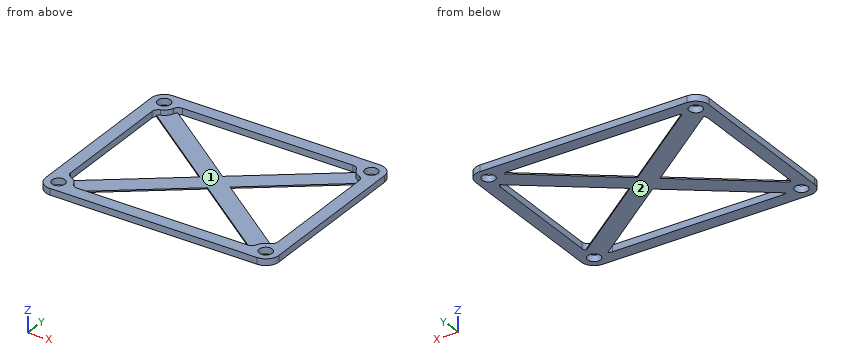
from build123d import *

# Parameters (mm, degrees)
SKETCH1_R           = 6.35
OUTLINE_DEPTH       = 6.35
FILLET2_R           = 12.7
BOSS_EXTRUDE1_DEPTH = 1.27
FILLET1_R           = 6.35


with BuildPart() as part:
    # Sketch1 → Outline (new body)
    with BuildSketch(Plane.XY):
        with BuildLine():
            Line((-101.6, 114.3), (101.6, 114.3))
            ThreePointArc((101.6, 114.3), (110.580256121, 110.580256121), (114.3, 101.6))
            Line((114.3, 101.6), (114.3, -66.802))
            Line((114.3, -66.802), (-114.3, -66.802))
            Line((-114.3, -66.802), (-114.3, 101.6))
            ThreePointArc((-114.3, 101.6), (-110.580256121, 110.580256121), (-101.6, 114.3))
        make_face()
        with Locations((-101.6, 101.6)):
            Circle(SKETCH1_R, mode=Mode.SUBTRACT)
        with Locations((101.6, 101.6)):
            Circle(SKETCH1_R, mode=Mode.SUBTRACT)
        with Locations((-101.6, -54.102)):
            Circle(SKETCH1_R, mode=Mode.SUBTRACT)
        with Locations(Location((101.6, -54.102, 0), (0, 0, 180))):
            Circle(SKETCH1_R, mode=Mode.SUBTRACT)
        with BuildLine():
            Line((-101.6, 88.9), (-101.6, -41.402))
            ThreePointArc((-101.6, -41.402), (-92.619743879, -45.121743879), (-88.9, -54.102))
            Line((-88.9, -54.102), (88.9, -54.102))
            ThreePointArc((88.9, -54.102), (92.619743879, -45.121743879), (101.6, -41.402))
            Line((101.6, -41.402), (101.6, 88.9))
            ThreePointArc((101.6, 88.9), (92.619743879, 92.619743879), (88.9, 101.6))
            Line((88.9, 101.6), (-88.9, 101.6))
            ThreePointArc((-88.9, 101.6), (-92.619743879, 92.619743879), (-101.6, 88.9))
        make_face(mode=Mode.SUBTRACT)
    extrude(amount=OUTLINE_DEPTH)

    # Fillet2
    fillet2_edges = [part.edges().sort_by_distance(p)[0] for p in [
        (114.3, -66.802, 3.175),
        (-114.3, -66.802, 3.175),
    ]]
    fillet(fillet2_edges, radius=FILLET2_R)

    # Sketch2 → Boss-Extrude1 (add)
    with BuildSketch(Plane(origin=(0, 0, 0), x_dir=(-1, 0, 0), z_dir=(0, 0, -1))):
        with BuildLine():
            Line((-101.6, 88.9), (-14.809147425, 23.749))
            Line((-14.809147425, 23.749), (-101.6, -41.402))
            ThreePointArc((-101.6, -41.402), (-92.619743879, -45.121743879), (-88.9, -54.102))
            Line((-88.9, -54.102), (0, 12.632266667))
            Line((0, 12.632266667), (88.9, -54.102))
            ThreePointArc((88.9, -54.102), (92.619743879, -45.121743879), (101.6, -41.402))
            Line((101.6, -41.402), (14.809147425, 23.749))
            Line((14.809147425, 23.749), (101.6, 88.9))
            ThreePointArc((101.6, 88.9), (92.619743879, 92.619743879), (88.9, 101.6))
            Line((88.9, 101.6), (0, 34.865733333))
            Line((0, 34.865733333), (-88.9, 101.6))
            ThreePointArc((-88.9, 101.6), (-92.619743879, 92.619743879), (-101.6, 88.9))
        make_face()
    extrude(amount=-BOSS_EXTRUDE1_DEPTH)

    # Fillet1
    # the kernel refuses this fillet: 6.35 mm, written as the material it adds along each edge
    with BuildSketch(Plane(origin=(101.6, 88.9, -11.881280605), x_dir=(0, -1, 0), z_dir=(0, 0, 1))) as fillet1_piece_1_section:
        with BuildLine():
            CenterArc((5.260512242, -6.35), FILLET1_R, 90, 70.528779366)
            ThreePointArc((-0.726325172, -4.233333333), (-0.182898292, -2.14759513), (0, 0))
            Line((0, 0), (5.260512242, 0))
        make_face()
    fillet1_piece_1 = extrude(amount=18.231280605, mode=Mode.PRIVATE)
    fillet1_piece_1 = split(fillet1_piece_1, bisect_by=Plane(origin=(101.237498755, 87.006858293, 0), z_dir=(0, 0, 1)), keep=Keep.TOP, mode=Mode.PRIVATE)
    add(fillet1_piece_1)
    with BuildSketch(Plane(origin=(88.9, 101.6, -11.881280605), x_dir=(-1, 0, 0), z_dir=(0, 0, 1))) as fillet1_piece_2_section:
        with BuildLine():
            CenterArc((5.260512242, 6.35), FILLET1_R, 199.471220634, 70.528779366)
            ThreePointArc((-0.726325172, 4.233333333), (-0.182898292, 2.14759513), (0, 0))
            Line((0, 0), (5.260512242, 0))
        make_face()
    fillet1_piece_2 = extrude(amount=18.231280605, mode=Mode.PRIVATE)
    fillet1_piece_2 = split(fillet1_piece_2, bisect_by=Plane(origin=(86.835808608, 101.33047194, 0), z_dir=(0, 0, 1)), keep=Keep.TOP, mode=Mode.PRIVATE)
    add(fillet1_piece_2)
    with BuildSketch(Plane(origin=(-101.6, 88.9, -11.881280605), x_dir=(0, -1, 0), z_dir=(0, 0, 1))) as fillet1_piece_3_section:
        with BuildLine():
            CenterArc((5.260512242, 6.35), FILLET1_R, 199.471220634, 70.528779366)
            ThreePointArc((-0.726325172, 4.233333333), (-0.182898292, 2.14759513), (0, 0))
            Line((0, 0), (5.260512242, 0))
        make_face()
    fillet1_piece_3 = extrude(amount=18.231280605, mode=Mode.PRIVATE)
    fillet1_piece_3 = split(fillet1_piece_3, bisect_by=Plane(origin=(-101.237498755, 87.006858293, 0), z_dir=(0, 0, 1)), keep=Keep.TOP, mode=Mode.PRIVATE)
    add(fillet1_piece_3)
    with BuildSketch(Plane(origin=(-88.9, 101.6, -11.881280605), x_dir=(1, 0, 0), z_dir=(0, 0, 1))) as fillet1_piece_4_section:
        with BuildLine():
            CenterArc((5.260512242, -6.35), FILLET1_R, 90, 70.528779366)
            ThreePointArc((-0.726325172, -4.233333333), (-0.182898292, -2.14759513), (0, 0))
            Line((0, 0), (5.260512242, 0))
        make_face()
    fillet1_piece_4 = extrude(amount=18.231280605, mode=Mode.PRIVATE)
    fillet1_piece_4 = split(fillet1_piece_4, bisect_by=Plane(origin=(-86.835808608, 101.33047194, 0), z_dir=(0, 0, 1)), keep=Keep.TOP, mode=Mode.PRIVATE)
    add(fillet1_piece_4)
    with BuildSketch(Plane(origin=(-101.6, -41.402, -11.881280605), x_dir=(0, 1, 0), z_dir=(0, 0, 1))) as fillet1_piece_5_section:
        with BuildLine():
            CenterArc((5.260512242, -6.35), FILLET1_R, 90, 70.528779366)
            ThreePointArc((-0.726325172, -4.233333333), (-0.182898292, -2.14759513), (0, 0))
            Line((0, 0), (5.260512242, 0))
        make_face()
    fillet1_piece_5 = extrude(amount=18.231280605, mode=Mode.PRIVATE)
    fillet1_piece_5 = split(fillet1_piece_5, bisect_by=Plane(origin=(-101.237498755, -39.508858293, 0), z_dir=(0, 0, 1)), keep=Keep.TOP, mode=Mode.PRIVATE)
    add(fillet1_piece_5)
    with BuildSketch(Plane(origin=(101.6, -41.402, -11.881280605), x_dir=(0, 1, 0), z_dir=(0, 0, 1))) as fillet1_piece_6_section:
        with BuildLine():
            CenterArc((5.260512242, 6.35), FILLET1_R, 199.471220634, 70.528779366)
            ThreePointArc((-0.726325172, 4.233333333), (-0.182898292, 2.14759513), (0, 0))
            Line((0, 0), (5.260512242, 0))
        make_face()
    fillet1_piece_6 = extrude(amount=18.231280605, mode=Mode.PRIVATE)
    fillet1_piece_6 = split(fillet1_piece_6, bisect_by=Plane(origin=(101.237498755, -39.508858293, 0), z_dir=(0, 0, 1)), keep=Keep.TOP, mode=Mode.PRIVATE)
    add(fillet1_piece_6)
    with BuildSketch(Plane(origin=(-88.9, -54.102, -11.881280605), x_dir=(1, 0, 0), z_dir=(0, 0, 1))) as fillet1_piece_7_section:
        with BuildLine():
            CenterArc((5.260512242, 6.35), FILLET1_R, 199.471220634, 70.528779366)
            ThreePointArc((-0.726325172, 4.233333333), (-0.182898292, 2.14759513), (0, 0))
            Line((0, 0), (5.260512242, 0))
        make_face()
    fillet1_piece_7 = extrude(amount=18.231280605, mode=Mode.PRIVATE)
    fillet1_piece_7 = split(fillet1_piece_7, bisect_by=Plane(origin=(-86.835808608, -53.83247194, 0), z_dir=(0, 0, 1)), keep=Keep.TOP, mode=Mode.PRIVATE)
    add(fillet1_piece_7)
    with BuildSketch(Plane(origin=(88.9, -54.102, -11.881280605), x_dir=(-1, 0, 0), z_dir=(0, 0, 1))) as fillet1_piece_8_section:
        with BuildLine():
            CenterArc((5.260512242, -6.35), FILLET1_R, 90, 70.528779366)
            ThreePointArc((-0.726325172, -4.233333333), (-0.182898292, -2.14759513), (0, 0))
            Line((0, 0), (5.260512242, 0))
        make_face()
    fillet1_piece_8 = extrude(amount=18.231280605, mode=Mode.PRIVATE)
    fillet1_piece_8 = split(fillet1_piece_8, bisect_by=Plane(origin=(86.835808608, -53.83247194, 0), z_dir=(0, 0, 1)), keep=Keep.TOP, mode=Mode.PRIVATE)
    add(fillet1_piece_8)


solid = part.part
For this review, take the finished solid that the model builds, in its own axes (mm). Face numbers are marked on the shaded views. Give positions to 0.01 mm unless a question says otherwise; leave off trailing zeros. Loops run counter-clockwise (first coordinate to the right, second up) from the corner with the lowest first, then second, coordinate; pieces in that order, holes last. Notation, with made-up numbers: M 37,-4.5 L 83,-4.5 A16 ccw 83,16.5 Z; hole C 51.25,14.25 d11. An arc over 180 degrees is marked long. Answer as a JSON object with one key per item and string values. Group by question number.
Q1. Mouldability with a two-part tool opening along X and no side actions: class the marked faces 1 and 2 as +X half, -X half, draft (parallel to the pull), parting line (faces both ways), or undercut.
Q2. Insertion check: P1, Ø7.5, axis at x = -101.6, y = -54.102, coming from the +Z side; P2, Ø5, axis at x = 71, y = -35, coming from the +Z side. Each pin has a flat end and moves straight along its axis. Give the tip position at first contact, or say it passes through.
Q3. Add section C-C on x = 72.5. Give the boundary of the cut face in (y, z), and give its area (3 significant figures).
Q4. Add section B-B on y = -21. Give the boundary of the cut face in (x, z).
Q5. For probe 1 along Y at (x, z) = (-66.5, 4.75); probe 2 along X at (y, z) = (64.5, 1.5); probe 3 along X at (y, z) = (100, 6), list the stretches that pass through material, from the lowest coordinate up. Write a range as [from, to].
Q6. Add section A-A on z = 3.5. Give the boundary of the cut face in (x, y).
Checked values:
{
 "1": {"face 1": "undercut", "face 2": "draft"},
 "2": {"P1": "through", "P2": "z = 1.27"},
 "3": {"outline": "M -66.8,0 L -54.1,0 L -54.1,6.35 L -66.8,6.35 Z; M -41.79,0 L -19.56,0 L -19.56,1.27 L -41.79,1.27 Z; M 67.06,0 L 89.29,0 L 89.29,1.27 L 67.06,1.27 Z; M 101.6,0 L 114.3,0 L 114.3,6.35 L 101.6,6.35 Z", "area": "218 mm²"},
 "4": {"outline": "M -114.3,0 L -101.6,0 L -101.6,6.35 L -114.3,6.35 Z; M -74.42,0 L -44.8,0 L -44.8,1.27 L -74.42,1.27 Z; M 44.8,0 L 74.42,0 L 74.42,1.27 L 44.8,1.27 Z; M 101.6,0 L 114.3,0 L 114.3,6.35 L 101.6,6.35 Z"},
 "5": {"probe 1": "[-66.8, -54.1], [101.6, 114.3]", "probe 2": "[-114.3, -101.6], [101.6, 114.3]", "probe 3": "[-114.3, -107.75], [-95.45, -87.85], [87.85, 95.45], [107.75, 114.3]"},
 "6": {"outline": "M -114.3,-54.1 A12.7 ccw -101.6,-66.8 L 101.6,-66.8 A12.7 ccw 114.3,-54.1 L 114.3,101.6 A12.7 ccw 101.6,114.3 L -101.6,114.3 A12.7 ccw -114.3,101.6 Z; hole C -101.6,-54.1 d12.7; hole C -101.6,101.6 d12.7; hole M -101.6,-36.14 A6.35 ccw -97.37,-42.13 A12.7 cw -89.63,-49.87 A6.35 ccw -83.64,-54.1 L 83.64,-54.1 A6.35 ccw 89.63,-49.87 A12.7 cw 97.37,-42.13 A6.35 ccw 101.6,-36.14 L 101.6,83.64 A6.35 ccw 97.37,89.63 A12.7 cw 89.63,97.37 A6.35 ccw 83.64,101.6 L -83.64,101.6 A6.35 ccw -89.63,97.37 A12.7 cw -97.37,89.63 A6.35 ccw -101.6,83.64 Z; hole C 101.6,-54.1 d12.7; hole C 101.6,101.6 d12.7"}
}
